Geometry: final body of the model. Coordinates: model frame, mm. A direction names the side the tool comes from. Give positions to 0.01 mm unless a question says otherwise; leave off trailing zeros. Write each loop counter-clockwise with the first axis right and the second up, starting at its lowest first coordinate (ties: lowest second). Pieces come first, ordered by that corner, then holes.
from build123d import *

# Parameters (mm, degrees)
BOSS_EXTRUDE1_DEPTH                     = 10
CBORE_FOR_M5_HEX_HEAD_BOLT1_D           = 5.3
CBORE_FOR_M5_HEX_HEAD_BOLT1_CBORE_D     = 12.24
CBORE_FOR_M5_HEX_HEAD_BOLT1_CBORE_DEPTH = 3.58
CHAMFER1_SIZE                           = 3


with BuildPart() as part:
    # Sketch1 → Boss-Extrude1 (new body)
    with BuildSketch(Plane.XY):
        with BuildLine():
            Line((-3.5, 9.367496998), (-3.5, -9.367496998))
            ThreePointArc((-3.5, -9.367496998), (10, 0), (-3.5, 9.367496998))
        make_face()
    extrude(amount=BOSS_EXTRUDE1_DEPTH)

    # CBORE for M5 Hex Head Bolt1 (through all)
    with Locations(Plane(origin=(0, 0, 0), x_dir=(-1, 0, 0), z_dir=(0, 0, -1))):
        with Locations((0, 0)):
            CounterBoreHole(CBORE_FOR_M5_HEX_HEAD_BOLT1_D / 2, CBORE_FOR_M5_HEX_HEAD_BOLT1_CBORE_D / 2, CBORE_FOR_M5_HEX_HEAD_BOLT1_CBORE_DEPTH)

    # Chamfer1
    chamfer1_edges = [part.edges().sort_by_distance(p)[0] for p in [
        (10, 0, 0),
    ]]
    chamfer(chamfer1_edges, length=CHAMFER1_SIZE)


solid = part.part
Q1. Pin query (flat end, axial travel): P1, Ø7.5, axis at x = 0.5, y = 0, coming from the -Z side; P2, Ø1.5, axis at x = 6.5, z = 8.5, coming from the +Y side; P3, Ø1, axis at x = 4.5, y = 4, coming from the -Z side; P4, Ø5, axis at x = 8.5, y = 4.5, coming from the -Z side. Return the tip coordinate at first contact, or that it passes through.
Filled sheet:
P1: stops at z = 3.58
P2: stops at y = 8.18
P3: stops at z = 0
P4: stops at z = 0.12
Q2. Access query for faces 4 (the flat face through (-3.5, 0, 6)), 5 (the flat face through (2.45, 1.45, 3.58)). Directions: +Z, -Z, +X, -X, +Y, -Y. A direction counts if a zero-diameter tool reaches every point of the face in a straight line with its end or side. Return the directions, or none.
Filled sheet:
face 4: +Z, -Z, -X, +Y, -Y
face 5: -Z
Q3. Section C-C on z = 6.75. Output: boundary loops of the cut face in (x, y), plus the area to 3 significant figures.
Filled sheet:
outline: (-3.5, -9.37) arc R10 ccw (long way) to (-3.5, 9.37) - close; hole circle Ø5.3 at (0, 0)
area: 204 mm2
Q4. Section A-A on x = 0. Output: boundary loops of the cut face in (y, z), plus the area to 3 significant figures.
Filled sheet:
outline: (-10, 3) - (-7, 0) - (-6.12, 0) - (-6.12, 3.58) - (-2.65, 3.58) - (-2.65, 10) - (-10, 10) - close; (2.65, 3.58) - (6.12, 3.58) - (6.12, 0) - (7, 0) - (10, 3) - (10, 10) - (2.65, 10) - close
area: 113 mm2
Q5. Pull-direction query (X, two-part tool) for faces 1 (the flat face through (3, 0, 10)), 2 (the cylindrical face through (6.117, 0.187, 1.765)), 3 (the cylindrical face through (10, 0, 6)); classes: released by +X, released by -X, zero draft, split by the parting line, or undercut.
Filled sheet:
face 1: zero draft
face 2: undercut
face 3: split by the parting line
Q6. Ray query, line 1 along Y through (x, z) = (0, 8.5); line 2 along Y through (x, z) = (0, 1.95); line 3 along X through (y, z) = (1, 6.25). Return the intervals inside material, ascending.
Filled sheet:
line 1: y = -10 to -2.65, 2.65 to 10
line 2: y = -8.95 to -6.12, 6.12 to 8.95
line 3: x = -3.5 to -2.45, 2.45 to 9.95
Q7. Section D-D on z = 1.25. Output: boundary loops of the cut face in (x, y), plus the area to 3 significant figures.
Filled sheet:
outline: (-3.5, -7.47) arc R8.25 ccw (long way) to (-3.5, 7.47) - (-3.5, 5.02) arc R6.12 cw (long way) to (-3.5, -5.02) - close
area: 63.7 mm2
Q8. Section B-B on y = 0. Output: boundary loops of the cut face in (x, z), plus the area to 3 significant figures.
Filled sheet:
outline: (-3.5, 3.58) - (-2.65, 3.58) - (-2.65, 10) - (-3.5, 10) - close; (2.65, 3.58) - (6.12, 3.58) - (6.12, 0) - (7, 0) - (10, 3) - (10, 10) - (2.65, 10) - close
area: 62.0 mm2
